The model under review builds one solid part; all positions refer to its coordinate system, in mm. Coordinates: 2 decimals unless noted, no trailing zeros. Loops run counter-clockwise (first coordinate to the right, second up) from the corner with the lowest first, then second, coordinate; pieces in that order, holes last. Notation, with made-up numbers: M 80.25,47.25 L 135.25,47.25 A16 ccw 135.25,62.25 Z; hole C 82.25,6.5 d7. An arc over 180 degrees is marked long. One line per item, written item: value.
Autodesk Inventor part; units mm, degrees
ref_plane "YZ Plane" through (0, 0, 0) normal (1, 0, 0) x (0, 1, 0)
ref_plane "XZ Plane" through (0, 0, 0) normal (0, 1, 0) x (-1, 0, 0)
ref_plane "XY Plane" through (0, 0, 0) normal (0, 0, 1) x (1, 0, 0)
sketch "Sketch1" plane through (0, 0, 0) normal (0, 0, 1) x (1, 0, 0)
  line L0 (0, 0) -> (-15, 0)
  line L1 (-15, 0) -> (-15, 5.9)
  line L2 (-15, 5.9) -> (0, 5.9)
  line L3 (0, 5.9) -> (0, 0)
  dimension "d0" = 5.9
  dimension "d1" = 15
extrude "Extrusion1" add sketch "Sketch1" along normal blind 4
sketch "Sketch2" plane through (-15, 5.9, 0) normal (0, 1, 0) x (1, 0, 0)
  circle A0 centre (12.5, -2) radius 0.8
  circle A1 centre (2.5, -2) radius 0.8
  line L0 (15, 0) -> (15, -4)
  line L1 (15, -4) -> (0, -4)
  dimension "d4" = 10
  dimension "d5" = 2.5
  dimension "d6" = 2
  dimension "d7" = 2
  dimension "d8" = 1.6
  dimension "d9" = 1.6
extrude "Extrusion2" cut sketch "Sketch2" against normal blind 8
sketch "Sketch3" plane through (0, 0, 0) normal (0, 0, -1) x (-1, 0, 0)
  line L0 (0, 0) -> (0, 5.9)
  line L1 (0, 0) -> (-10, 0)
  line L2 (-10, 0) -> (-10, 5.9)
  line L3 (-10, 5.9) -> (0, 5.9)
  line L4 (0, 5.9) -> (0, 0)
  dimension "d12" = 10
extrude "Extrusion3" add sketch "Sketch3" against normal blind 4
sketch "Sketch4" plane through (0, 0, 0) normal (0, 0, -1) x (-1, 0, 0)
  line L0 (3.3, 5.9) -> (3.3, 0)
  line L1 (1.7, 5.9) -> (1.7, 0)
  circle A0 centre (-3, 1.9) radius 0.8
  circle A1 centre (-7, 1.9) radius 0.8
  line L2 (-10, 5.9) -> (15, 5.9)
  line L3 (15, 0) -> (-10, 0)
  line L4 (-10, 5.9) -> (-10, 0)
  point P0 (0, 0)
  dimension "d15" = 1.6
  dimension "d16" = 5.9
  dimension "d17" = 4
  dimension "d18" = 4
  dimension "d19" = 4
  dimension "d20" = 3
  dimension "d21" = 1.6
  dimension "d22" = 1.6
extrude "Extrusion4" cut sketch "Sketch4" against normal blind 4 contours A0 | A1
equation "\"d7\" = d6"
equation "\"d18\" = d17"
equation "\"d21\" = d15"
equation "\"d22\" = d15"
properties part number "AngleScrewBlocActuator"
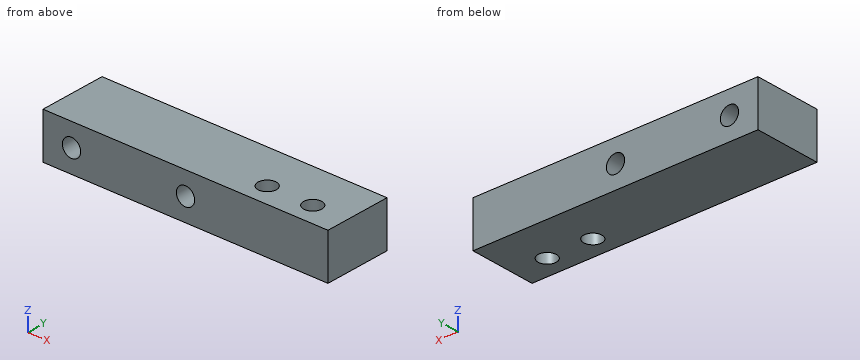
(1) Add section C-C on x = 3. State the section outline as (y, z) points, then the cut area to 3 significant figures.
Checks:
outline: M 0,0 L 1.1,0 L 1.1,4 L 0,4 Z; M 2.7,0 L 5.9,0 L 5.9,4 L 2.7,4 Z
area: 17.2 mm^2
(2) Add section D-D on y = 4.85. State the section outline as (x, z) points, then the cut area to 3 significant figures.
Checks:
outline: M -15,0 L 10,0 L 10,4 L -15,4 Z; hole C -12.5,2 d1.6; hole C -2.5,2 d1.6
area: 96.0 mm^2
(3) Add section B-B on y = 1.9. State the section outline as (x, z) points, then the cut area to 3 significant figures.
Checks:
outline: M -15,0 L 2.2,0 L 2.2,4 L -15,4 Z; M 3.8,0 L 6.2,0 L 6.2,4 L 3.8,4 Z; M 7.8,0 L 10,0 L 10,4 L 7.8,4 Z; hole C -12.5,2 d1.6; hole C -2.5,2 d1.6
area: 83.2 mm^2
(4) Insertion check: pin 1 Ø1.4 at (x, y) = (3, 1.9) entering from +Z. The pin has a flat end and moves straight along its axis. Give the tip position at first contact, or say it passes through.
Checks:
pin 1: through
(5) To check wall thickness, follow L1, parallel to X at y = 2.9, z = 2; L2, parallel to Y at x = 7, z = 2.6; L3, parallel to X at y = 2.6, z = 3. State the ranges of each line that lie inside material, in increasing order. Write a range as [from, to].
Checks:
L1: [-15, -13.3], [-11.7, -3.3], [-1.7, 10]
L2: [0, 1.1], [2.7, 5.9]
L3: [-15, 2.61], [3.39, 6.61], [7.39, 10]
(6) Add section A-A on z = 2. State the section outline as (x, y) points, then the cut area to 3 significant figures.
Checks:
outline: M -15,0 L -13.3,0 L -13.3,5.9 L -15,5.9 Z; M -11.7,0 L -3.3,0 L -3.3,5.9 L -11.7,5.9 Z; M -1.7,0 L 10,0 L 10,5.9 L -1.7,5.9 Z; hole C 3,1.9 d1.6; hole C 7,1.9 d1.6
area: 125 mm^2
